```python
from build123d import *

# Parameters (mm, degrees)
SKETCH2_R          = 31.732831761
CUT_EXTRUDE1_DEPTH = 26.78316707
SKETCH3_R          = 11.120214541
SKETCH3_R_2        = 5.08
CUT_EXTRUDE2_DEPTH = 12.7
CUT_EXTRUDE2_DRAFT = -3
FILLET1_R          = 0.635


with BuildPart() as part:
    # Sketch1 → Revolve1 (revolve)
    with BuildSketch(Plane(origin=(0, 0, 0), x_dir=(0, 0, -1), z_dir=(1, 0, 0)), mode=Mode.PRIVATE) as revolve1_sk:
        Polygon((3.175, 3.175), (3.81, 3.81), (4.318, 3.81), (4.953, 3.175), (6.5405, 3.175), (7.5565, 4.191), (9.0805, 4.191), (9.0805, 4.064), (13.954125, 4.064), (13.954125, 4.191), (15.478125, 4.191), (15.478125, 14.36586369), (31.353125, 14.36586369), (31.353125, 0), (12.7, 0), (12.7, 1.5875), (0, 1.5875), (0, 3.175), align=None)
    revolve(revolve1_sk.sketch.rotate(Axis((0, 0, -12.7), (0, 0, -1)), 180), axis=Axis((0, 0, -12.7), (0, 0, -1)))

    # Sketch2 → Cut-Extrude1 (cut, through all)
    with BuildSketch(Plane(origin=(0, 0, -15.478125), x_dir=(-1, 0, 0), z_dir=(0, 0, -1))):
        Circle(SKETCH2_R)
        Polygon((7.332348419, 0), (3.666174209, 6.35), (-3.666174209, 6.35), (-7.332348419, 0), (-3.666174209, -6.35), (3.666174209, -6.35), align=None, mode=Mode.SUBTRACT)
    extrude(amount=CUT_EXTRUDE1_DEPTH, mode=Mode.SUBTRACT)


with BuildPart() as cut_extrude2_tool:
    # Sketch3 → Cut-Extrude2 (with draft: the straight prism first)
    with BuildSketch(Plane(origin=(0, 0, -31.353125), x_dir=(-1, 0, 0), z_dir=(0, 0, -1))):
        Circle(SKETCH3_R)
        Circle(SKETCH3_R_2, mode=Mode.SUBTRACT)
    extrude(amount=-CUT_EXTRUDE2_DEPTH)
    # Cut-Extrude2: the draft: its side faces are tilted about the plane it starts from
    cut_extrude2_sides = [cut_extrude2_tool.faces().sort_by_distance(p)[0] for p in [
        (11.120214541, 0, -25.003125),
        (5.08, 0, -25.003125),
    ]]
    draft(cut_extrude2_sides, Plane(origin=(0, 0, -31.353125), x_dir=(-1, 0, 0), z_dir=(0, 0, -1)), CUT_EXTRUDE2_DRAFT)


with BuildPart() as part_1:
    add(part.part)

    # Cut-Extrude2: cut by cut_extrude2_tool
    add(cut_extrude2_tool.part, mode=Mode.SUBTRACT)

    # Fillet1
    fillet1_edges = [part_1.edges().sort_by_distance(p)[0] for p in [
        (0, 3.175, 0),
        (-3.666174209, -6.35, -17.065625),
        (3.666174209, -6.35, -17.065625),
        (7.332348419, 0, -17.065625),
        (3.666174209, 6.35, -17.065625),
        (-3.666174209, 6.35, -17.065625),
        (-7.332348419, 0, -17.065625),
    ]]
    fillet(fillet1_edges, radius=FILLET1_R)


solid = part_1.part
```
Source: CAD feature listing. Evaluate the final solid. Frame: model axes, mm. A direction names the side the tool comes from. Give positions to 0.01 mm unless a question says otherwise; leave off trailing zeros. Order: outer loops, then holes, each group sorted by start corner. A loop starts at its lowest first (then second) coordinate and runs counter-clockwise, first axis right, second up. Notation, with made-up numbers: (60.5, -14.75) -> (92.5, -14.75) arc R9 ccw to (92.5, -9.75) -> close; hole circle Ø7 at (-28, 38.5). An arc over 180 degrees is marked (long way). Use a Markdown table: item, result.
Q1. Section B-B (z = -25). Return the cut outline in (x, y), and give its area (3 significant figures).
A:
| item | result |
|---|---|
| outline | circle Ø10.83 at (0, 0) |
| area | 92.0 mm^2 |
Q2. Section C-C (z = -20.5). Return the cut outline in (x, y), and give its area (3 significant figures).
A:
| item | result |
|---|---|
| outline | circle Ø11.3 at (0, 0) |
| area | 100 mm^2 |
Q3. Material intervals for line 1 (X direction, y = 0, z = -6) (1 decimal); line 2 (X direction, y = 0, z = -10); line 3 (Z direction, x = -5.75, y = -1.25), sorted ascending. Write a range as [from, to].
A:
| item | result |
|---|---|
| line 1 | [-3.2, -1.6], [1.6, 3.2] |
| line 2 | [-4.06, -1.59], [1.59, 4.06] |
| line 3 | [-18.65, -15.48] |
Q4. Access query for faces 1 (the face through (1, 6, -18.653)), 2 (the face through (-3.3, -2.9, -15.478)), 3 (the face through (2.8, -1.5, -5.8)). Directions: +Z, -Z, +X, -X, +Y, -Y. A direction counts if a zero-diameter tool reaches every point of the face in a straight line with its end or side. Return the directions, or none.
A:
| item | result |
|---|---|
| face 1 | -Z |
| face 2 | +Z |
| face 3 | none |
Q5. Section A-A (z = -8). Return the cut outline in (x, y) (1 decimal), and give its area (3 significant figures).
A:
| item | result |
|---|---|
| outline | circle Ø8.4 at (0, 0); hole circle Ø3.2 at (0, 0) |
| area | 47.3 mm^2 |
Q6. Pull-direction query (X, two-part tool) for faces 4 (the face through (0, 0, -12.7)), 5 (the face through (2.8, -1.5, -1.9)), 6 (the face through (0, 0, -31.353)); classes: +X half, -X half, draft (parallel to the pull), parting line (faces both ways), or undercut.
A:
| item | result |
|---|---|
| face 4 | undercut |
| face 5 | parting line |
| face 6 | draft |
Q7. First-contact query: P1, Ø3, axis at x = -0.5, z = -20.5, coming from the +Y side; P2, Ø1.6, axis at x = -0.5, y = 0.5, coming from the +Z side; P3, Ø1.5, axis at x = -5.5, z = -17.5, coming from the -Y side; P4, Ø3, axis at x = -5.5, y = 1.5, coming from the -Z side. Flat tips, straight axial feed; report the tip coordinate or a pass-through.
A:
| item | result |
|---|---|
| P1 | y = 5.72 |
| P2 | z = -12.7 |
| P3 | y = -4.47 |
| P4 | z = -31.35 |
